Build history of the part. All positions in model axes, mm. A direction names the side the tool comes from. Coordinates: 2 decimals unless noted, no trailing zeros. Loops run counter-clockwise (first coordinate to the right, second up) from the corner with the lowest first, then second, coordinate; pieces in that order, holes last. Notation, with made-up numbers: (45, -19) -> (62, -19) arc R22 cw to (62, 13) -> close; hole circle Ø9 at (-22.5, 48). An arc over 180 degrees is marked (long way). One line per item, written item: value. Start each with the question number.
```python
from build123d import *

# Parameters (mm, degrees)
F1_DEPTH = 30


with BuildPart() as f1:
    # F0 (on Front) → F1 (new body)
    with BuildSketch(Plane.XZ):
        with BuildLine():
            ThreePointArc((43.9601876184, -40.8350572983), (55.8462678122, -21.9361430395), (60, 0))
            ThreePointArc((60, 0), (59.3271357487, 8.9605225212), (57.3236345382, 17.7200711998))
            ThreePointArc((57.3236345382, 17.7200711998), (35.6145737586, 48.286666234), (0, 60))
            Line((0, 60), (-6.1995762038, 59.678850985))
            ThreePointArc((-6.1995762038, 59.678850985), (-45.9961514375, 38.5273156726), (-59.8412528078, -4.3617040695))
            ThreePointArc((-59.8412528078, -4.3617040695), (-45.749304661, -38.8201123522), (-14.0443202253, -58.3331558328))
            ThreePointArc((-14.0443202253, -58.3331558328), (13.2837711962, -58.5110367607), (37.8560106248, -46.5502143881))
            Line((37.8560106248, -46.5502143881), (43.9601876184, -40.8350572983))
        make_face()
        with BuildLine():
            ThreePointArc((22.2544550068, -8.9855012298), (-23.9879968678, -0.7589507694), (21.6419337451, 10.3743290757))
            Line((21.6419337451, 10.3743290757), (34, 11.0144987702))
            Line((34, 11.0144987702), (34, -8.9855012298))
            Line((34, -8.9855012298), (22.2544550068, -8.9855012298))
        make_face(mode=Mode.SUBTRACT)
        with BuildLine():
            ThreePointArc((57.3236345382, 17.7200711998), (59.3271357487, 8.9605225212), (60, 0))
            ThreePointArc((60, 0), (55.8462678122, -21.9361430395), (43.9601876184, -40.8350572983))
            Line((43.9601876184, -40.8350572983), (141.2785439355, 50.2811889465))
            ThreePointArc((141.2785439355, 50.2811889465), (117.6128786081, 46.9029106044), (96.7146143427, 58.5106248772))
            Line((96.7146143427, 58.5106248772), (57.3236345382, 17.7200711998))
        make_face()
        with BuildLine():
            ThreePointArc((0, 60), (35.6145737586, 48.286666234), (57.3236345382, 17.7200711998))
            Line((57.3236345382, 17.7200711998), (96.7146143427, 58.5106248772))
            ThreePointArc((96.7146143427, 58.5106248772), (86.9363192525, 84.7896597627), (98.1158209388, 110.5038867865))
            Line((98.1158209388, 110.5038867865), (-6.1995762038, 59.678850985))
            ThreePointArc((-6.1995762038, 59.678850985), (-3.1039443373, 59.9196589572), (0, 60))
        make_face()
        with BuildLine():
            ThreePointArc((37.8560106248, -46.5502143881), (41.0077837597, -43.7991058255), (43.9601876184, -40.8350572983))
            Line((43.9601876184, -40.8350572983), (37.8560106248, -46.5502143881))
        make_face()
        with BuildLine():
            Line((-6.1995762038, 59.678850985), (0, 60))
            ThreePointArc((0, 60), (-3.1039443373, 59.9196589572), (-6.1995762038, 59.678850985))
        make_face()
        with BuildLine():
            ThreePointArc((98.1158209388, 110.5038867865), (86.9363192525, 84.7896597627), (96.7146143427, 58.5106248772))
            ThreePointArc((96.7146143427, 58.5106248772), (117.6128786081, 46.9029106044), (141.2785439355, 50.2811889465))
            ThreePointArc((141.2785439355, 50.2811889465), (156.3471806883, 64.105109847), (161.9227087237, 83.779410083))
            ThreePointArc((161.9227087237, 83.779410083), (138.9096288254, 118.3681242246), (98.1158209388, 110.5038867865))
        make_face()
        with BuildLine():
            ThreePointArc((139.4227087237, 83.779410083), (129.1669853294, 69.5494473463), (112.4237967918, 74.7779595082))
            ThreePointArc((112.4237967918, 74.7779595082), (119.678432118, 98.0093728198), (139.4227087237, 83.779410083))
        make_face(mode=Mode.SUBTRACT)
        with BuildLine():
            ThreePointArc((-59.8412528078, -4.3617040695), (-45.9961514375, 38.5273156726), (-6.1995762038, 59.678850985))
            Line((-6.1995762038, 59.678850985), (-232.1886784593, 47.9722156929))
            Line((-232.1886784593, 47.9722156929), (-231.2155919095, 29.1874026098))
            Line((-231.2155919095, 29.1874026098), (-193.7155919095, 29.1874026098))
            ThreePointArc((-193.7155919095, 29.1874026098), (-174.663504004, 16.9450214035), (-166.9900822915, -4.3617040695))
            Line((-166.9900822915, -4.3617040695), (-59.8412528078, -4.3617040695))
        make_face()
        with BuildLine():
            Line((-232.5, -58.3331558328), (-14.0443202253, -58.3331558328))
            ThreePointArc((-14.0443202253, -58.3331558328), (-45.749304661, -38.8201123522), (-59.8412528078, -4.3617040695))
            Line((-59.8412528078, -4.3617040695), (-166.9900822915, -4.3617040695))
            ThreePointArc((-166.9900822915, -4.3617040695), (-174.663504004, -26.9861874019), (-195, -39.5231558328))
            Line((-195, -39.5231558328), (-232.5, -39.5231558328))
            Line((-232.5, -39.5231558328), (-232.5, -58.3331558328))
        make_face()
    extrude(amount=F1_DEPTH)


solid = f1.part
```
Item 1: Band-saw the part on C-C, the plane y = -17.75. List the corners of the cut face in (x, z), and give its area (3 significant figures).
Item 2: Tool access for faces 4 (the face through (-38, 0, 12)), 5 (the face through (27.73, -14.79, 10.69)), 6 (the face through (-125, -15, -58.333)), 7 (the face through (91.938, -14.79, 4.085)), 8 (the face through (-213, -15, -39.523)): list every direction of +Z, -Z, +X, -X, +Y, -Y with a clear straight run to the whole face (end or side of a thin tool).
Item 3: Band-saw the part on A-A, the plane x = 130.5. List the corners of the cut face in (y, z), and give its area (4 significant figures).
Item 4: Band-saw the part on D-D, the plane x = 52.5. List the corners of the cut face in (y, z), and give its area (3 significant figures).
Item 5: Drop flat-ended pins along their axis: pin 1 Ø13 at (x, y) = (28, -22) entering from +Z; pin 2 Ø9 at (x, y) = (-121.5, -17.5) entering from -Z; pin 3 Ø8 at (y, z) = (-17, 3) entering from -X. Give the stop position or say it passes through.
Item 6: Two-plate mould, pull along X, no slides. Class faces 1 (the face through (46.69, -14.79, 85.45)), 2 (the face through (-23.94, -14.79, -1.67)), 3 (the face through (-38, -30, 12)): +X half, -X half, draft (parallel to the pull), parting line (faces both ways), or undercut.
Item 7: Band-saw the part on B-B, the plane z = 91. List the corners of the cut face in (x, y).
Item 8: Probe probe 1 along X at (y, z) = (-6.75, 87); probe 2 along X at (y, z) = (-12.75, 0); probe 3 along Z at (x, y) = (0, -12.5). List the from-to ranges inside material, lowest first.
Worked out:
1. outline: (-232.5, -58.33) -> (-14.04, -58.33) arc R60 ccw to (43.96, -40.84) -> (141.28, 50.28) arc R37.5 ccw (long way) to (98.12, 110.5) -> (-6.2, 59.68) -> (-232.19, 47.97) -> (-231.22, 29.19) -> (-193.72, 29.19) arc R35.25 cw to (-195, -39.52) -> (-232.5, -39.52) -> close; hole (21.64, 10.37) arc R24 ccw (long way) to (22.25, -8.99) -> (34, -8.99) -> (34, 11.01) -> close; hole circle Ø30 at (124.42, 83.78)
1. area: 35,900 mm²
2. face 4: +Z, -Z, +X, -X, +Y
2. face 5: +Y, -Y
2. face 6: -Z, -X, +Y, -Y
2. face 7: -Z, +X, +Y, -Y
2. face 8: -X, +Y, -Y
3. outline: (-30, 40.19) -> (0, 40.19) -> (0, 70.07) -> (-30, 70.07) -> close; (-30, 97.49) -> (0, 97.49) -> (0, 120.78) -> (-30, 120.78) -> close
3. area: 1,595 mm²
4. outline: (-30, -32.84) -> (0, -32.84) -> (0, 88.28) -> (-30, 88.28) -> close
4. area: 3,630 mm²
5. pin 1: stops at z = 79.51
5. pin 2: stops at z = -58.33
5. pin 3: stops at x = -169.1
6. face 1: -X half
6. face 2: undercut
6. face 3: draft
7. outline: (58.09, -30) -> (111.27, -30) -> (111.27, 0) -> (58.09, 0) -> close; (137.57, -30) -> (161.22, -30) -> (161.22, 0) -> (137.57, 0) -> close
8. probe 1: x = 49.88 to 109.77, 139.07 to 161.78
8. probe 2: x = -167.34 to -24, 34 to 87.57
8. probe 3: z = -60 to -24, 24 to 62.7
